```python
from build123d import *

# Parameters (mm, degrees)
F1_DEPTH = 0.635
F2_SIZE  = 0.63499
F3_DEPTH = 3.175
F4_SIZE  = 0.63499


# Not quite as in the source:
# - a fillet or chamfer is up to 0.001 mm smaller than in the source, because OpenCascade refuses the exact size


with BuildPart() as f1:
    # F0 (on Front) → F1 (new body, symmetric)
    with BuildSketch(Plane.XZ):
        Polygon((12.7, 177.8), (0, 203.2), (-12.7, 177.8), (-12.7, 0), (-6.35, -3.175), (-6.35, -50.8), (0, -50.8), (6.35, -50.8), (6.35, -3.175), (12.7, 0), align=None)
        Polygon((-6.35, 177.8), (0, 190.5), (6.35, 177.8), (6.35, 3.175), (0, 0), (-6.35, 3.175), align=None, mode=Mode.SUBTRACT)
    extrude(amount=F1_DEPTH, both=True)

    # F2 (size 0.635 in the source; OpenCascade refuses exactly that, so slightly less here)
    f2_edges = [f1.edges().sort_by_distance(p)[0] for p in [
        (12.7, -0.635, 88.9),
        (6.35, -0.635, 190.5),
        (-6.35, -0.635, 190.5),
        (-12.7, -0.635, 88.9),
        (-9.525, -0.635, -1.5875),
        (9.525, -0.635, -1.5875),
        (-9.525, 0.635, -1.5875),
        (9.525, 0.635, -1.5875),
        (-12.7, 0.635, 88.9),
        (12.7, 0.635, 88.9),
        (-6.35, 0.635, 190.5),
        (6.35, 0.635, 190.5),
    ]]
    chamfer(f2_edges, length=F2_SIZE)

    # F0 (on Front) → F3 (join, symmetric)
    with BuildSketch(Plane.XZ):
        Polygon((0, -50.8), (-6.35, -50.8), (-29.0684506514, -39.4407746743), (-29.0684506514, -45.7907746743), (-6.35, -57.15), (-3.175, -57.15), (0, -57.15), (3.175, -57.15), (6.35, -57.15), (29.0684506514, -45.7907746743), (29.0684506514, -39.4407746743), (6.35, -50.8), align=None)
    extrude(amount=F3_DEPTH, both=True)

    # F4 (size 0.635 in the source; OpenCascade refuses exactly that, so slightly less here)
    f4_edges = [f1.edges().sort_by_distance(p)[0] for p in [
        (6.35, -0.635, 90.4875),
        (-6.35, -0.635, 90.4875),
        (3.175, -0.635, 1.5875),
        (-3.175, -0.635, 1.5875),
        (-3.175, -0.635, 184.15),
        (3.175, -0.635, 184.15),
        (3.175, 0.635, 184.15),
        (-3.175, 0.635, 184.15),
        (-6.35, 0.635, 90.4875),
        (6.35, 0.635, 90.4875),
        (-3.175, 0.635, 1.5875),
        (3.175, 0.635, 1.5875),
    ]]
    chamfer(f4_edges, length=F4_SIZE)


solid = f1.part
```
Source: CAD feature listing. Evaluate the final solid. Frame: model axes, mm. A direction names the side the tool comes from. Give positions to 0.01 mm unless a question says otherwise; leave off trailing zeros. Loops run counter-clockwise (first coordinate to the right, second up) from the corner with the lowest first, then second, coordinate; pieces in that order, holes last. Notation, with made-up numbers: (-36, 56.25) - (15, 56.25) arc R13 ccw to (15, 81.25) - close; hole circle Ø7 at (-14.75, 38). An arc over 180 degrees is marked (long way). Use CSV: the item, a comma, the result in double quotes.
1) Cut plane D-D (x = 20). Output: boundary loops of the cut face in (y, z) (3 decimals).
Worked out:
outline,"(-3.175, -50.325) - (3.175, -50.325) - (3.175, -43.975) - (-3.175, -43.975) - close"
2) Cut plane C-C (z = -35). Output: boundary loops of the cut face in (x, y) (3 decimals), and give its area (3 significant figures).
Worked out:
outline,"(-6.35, -0.635) - (6.35, -0.635) - (6.35, 0.635) - (-6.35, 0.635) - close"
area,"16.1 mm^2"
3) Cut plane B-B (y = -2). Output: boundary loops of the cut face in (x, z).
Worked out:
outline,"(-29.07, -45.79) - (-6.35, -57.15) - (6.35, -57.15) - (29.07, -45.79) - (29.07, -39.44) - (6.35, -50.8) - (-6.35, -50.8) - (-29.07, -39.44) - close"
4) Pin query (flat end, axial travel): P1, Ø0.6, axis at y = 0, z = -18, coming from the -X side; P2, Ø2, axis at x = -11.5, z = 16, coming from the +Y side (3 decimals); P3, Ø0.8, axis at x = 1, y = -2, coming from the +Z side. Return the tip coordinate at first contact, or that it passes through.
Worked out:
P1,"stops at x = -6.35"
P2,"stops at y = 0.635"
P3,"stops at z = -50.8"
5) Line query: line 1 (Y direction, x = 11, z = 68) (3 decimals); line 2 (Z direction, x = 9.5, y = -0.5) (3 decimals); line 3 (Z direction, x = -6, y = -0.75). Output: solid intervals per line, ascending.
Worked out:
line 1,"y = -0.635 to 0.635"
line 2,"z = -55.575 to -49.225, -1.041 to 183.082"
line 3,"z = -57.15 to -50.8"
6) Mould query, pull axis X, two halves, no side actions, for faces 1 (the flat face through (0, -3.175, -51)), 2 (the flat face through (6.15, -0.32, 190.18)), 3 (the flat face through (3.156, -0.313, 184.889)). Classes: +X half, -X half, draft (parallel to the pull), parting line (faces both ways), or undercut.
Worked out:
face 1,"draft"
face 2,"+X half"
face 3,"undercut"
7) Set-up query: faces 4 (the flat face through (-3.25, 0.31, 184.69)), 5 (the flat face through (6.15, 0.32, 190.18)). Return all of +Z, -Z, +X, -X, +Y, -Y with unobstructed straight access to the full face (end or side cutting, diameter ignored); none if empty.
Worked out:
face 4,"+Y"
face 5,"+Z, +X, +Y"
